Can you work these out from the model? Positions are in its coordinate system, mm. A direction names the side the tool comes from. Round coordinates to 2 decimals unless told otherwise and drop trailing zeros. Write each loop counter-clockwise with the first axis right and the second up, starting at its lowest first coordinate (ties: lowest second). Pieces come first, ordered by that corner, then holes. Notation, with made-up numbers: (19.5, 28.25) -> (45.5, 28.25) arc R10 cw to (45.5, 42.25) -> close; hole circle Ø2 at (69.25, 59). An arc over 180 degrees is marked (long way). Write item = value, one per line. Start each with the question number.
1) Imagine slicing it at C-C, the plane y = -6.75. Please give me the cut outline in (x, z) (3 decimals), then the cut area to 3 significant figures.
2) Thinking about a two-plate mould opening in Z: for faces 3 (the face through (-49, -5, 0)), 4 (the face through (57, 0, -22)), 5 (the face through (33.69, -4.93, -115.06)), 6 (the face through (32.827, -4.93, 65.213)), which applies, +Z half, -Z half, draft (parallel to the pull), parting line (faces both ways), or undercut?
3) Imagine slicing it at B-B, the plane z = 75. Please give me the cut outline in (x, y) (3 decimals).
4) If I drill on line 1 (Z direction, x = -39, y = -3); line 2 (X direction, y = -0.75, z = -126.5); line 3 (X direction, y = -5.5, z = 10), over which ranges is the centre line in solid material (lowest first)?
5) Imagine slicing it at A-A, the plane x = 35. Please give me the cut outline in (y, z) (3 decimals).
6) For faces 1 (the face through (57, -10, -22)), 2 (the face through (0, -5, 51)), which set-ups out of +Z, -Z, +X, -X, +Y, -Y let a thin tool reach every point of the face, with its end or its side?
7) I'm going to push flat-ended pins straight in: pin 1 (1 mm diameter, centred on y = -4, z = 17, fed in from -X); pin 2 (3 mm diameter, centred on x = 182.5, y = -1.5, fed in from +Z); pin 3 (3 mm diameter, centred on y = -2.5, z = -102.5, fed in from +X); pin 4 (1 mm diameter, centred on x = 69, z = -120, fed in from +Y). Where does each tip first touch, or does it pass through?
8) Imagine slicing it at D-D, the plane x = -49. Please give me the cut outline in (y, z).
from build123d import *

# Parameters (mm, degrees)
F0_R     = 10.025
F1_DEPTH = 10


with BuildPart() as f1:
    # F0 (on Front) → F1 (new body)
    with BuildSketch(Plane.XZ):
        with BuildLine():
            Line((0, 100), (0, 0))
            Line((0, 0), (-100, 0))
            Line((-100, 0), (-100, -150))
            Line((-100, -150), (59.497475, -150))
            Line((59.497475, -150), (218.847763, 9.350288))
            ThreePointArc((218.847763, 9.350288), (122.139295, 85.372867), (0, 100))
        make_face()
        with Locations((35, -125)):
            Circle(F0_R, mode=Mode.SUBTRACT)
        with Locations((35, 75)):
            Circle(F0_R, mode=Mode.SUBTRACT)
        with Locations((176.421356, 16.421356)):
            Circle(F0_R, mode=Mode.SUBTRACT)
        with Locations((111.536686, 59.775907)):
            Circle(F0_R, mode=Mode.SUBTRACT)
    extrude(amount=F1_DEPTH)


solid = f1.part
Reported:
q1.outline = (-100, -150) -> (59.497, -150) -> (218.848, 9.35) arc R227.706 ccw to (0, 100) -> (0, 0) -> (-100, 0) -> close; hole circle Ø20.05 at (35, -125); hole circle Ø20.05 at (35, 75); hole circle Ø20.05 at (111.537, 59.776); hole circle Ø20.05 at (176.421, 16.421)
q1.area = 51,200 mm²
q2.face_3 = +Z half
q2.face_4 = draft
q2.face_5 = undercut
q2.face_6 = undercut
q3.outline = (0, -10) -> (24.975, -10) -> (24.975, 0) -> (0, 0) -> close; (45.025, -10) -> (143.858, -10) -> (143.858, 0) -> (45.025, 0) -> close
q4.line_1 = -150 to 0
q4.line_2 = -100 to 25.09, 44.91 to 83
q4.line_3 = 0 to 168.72, 184.12 to 218.37
q5.outline = (-10, -150) -> (0, -150) -> (0, -135.025) -> (-10, -135.025) -> close; (-10, -114.975) -> (0, -114.975) -> (0, 64.975) -> (-10, 64.975) -> close; (-10, 85.025) -> (0, 85.025) -> (0, 102.706) -> (-10, 102.706) -> close
q6.face_1 = +Z, -Z, +X, -X, -Y
q6.face_2 = +Z, -X, +Y, -Y
q7.pin_1 = 0
q7.pin_2 = 49.74
q7.pin_3 = 108.5
q7.pin_4 = 0
q8.outline = (-10, -150) -> (0, -150) -> (0, 0) -> (-10, 0) -> close
